from build123d import *

# Parameters (mm, degrees)
BOSS_EXTRUDE1_DEPTH     = 12.7
FILLET1_R               = 9.525
CUT_EXTRUDE3_DEPTH      = 171.371755619
CUT_EXTRUDE3_DEPTH_BACK = 171.371755619
SKETCH2_R               = 5.55625


with BuildPart() as part:
    # Sketch1 → Boss-Extrude1 (new body)
    with BuildSketch(Plane(origin=(0, 0, 0), x_dir=(0, 0, -1), z_dir=(1, 0, 0))):
        Polygon((0, 152.4), (-91.160761442, 0), (91.160761442, 0), align=None)
    extrude(amount=BOSS_EXTRUDE1_DEPTH)

    # Fillet1
    fillet1_edges = [part.edges().sort_by_distance(p)[0] for p in [
        (6.35, 152.4, 0),
    ]]
    fillet(fillet1_edges, radius=FILLET1_R)

    # Sketch2 → Cut-Extrude3 (cut, two sides: drawn at the far end of the back side and taken through both)
    with BuildSketch(Plane(origin=(0, 0, 0), x_dir=(0, 0, -1), z_dir=(1, 0, 0)).offset(-CUT_EXTRUDE3_DEPTH_BACK)):
        with Locations((0, 106.68)):
            Circle(SKETCH2_R)
    extrude(amount=CUT_EXTRUDE3_DEPTH + CUT_EXTRUDE3_DEPTH_BACK, mode=Mode.SUBTRACT)


solid = part.part
Here's how the part is built. I have some questions about the finished solid (model axes, mm). Coordinates: 2 decimals unless noted, no trailing zeros. Loops run counter-clockwise (first coordinate to the right, second up) from the corner with the lowest first, then second, coordinate; pieces in that order, holes last.
1. Imagine slicing it at A-A, the plane z = 0. Please give me the cut outline in (x, y).
2. I need wall thicknesses on L1, parallel to Y at x = 8.25, z = 0; L2, parallel to Z at x = 11.5, y = 107; L3, parallel to Z at x = 3, y = 106.5. Which ranges of each line are inside material? Lowest first, please.
3. Imagine slicing it at C-C, the plane y = 106.68. Please give me the cut outline in (x, z), and give its area (3 significant figures).
4. For P1, Ø1, axis at x = 7, y = 58, coming from the +Z side; P2, Ø3, axis at x = 6.5, z = 56, coming from the +Y side; P3, Ø6, axis at x = 4, z = 35, coming from the +Y side, each with a flat end and sliding along its axis, tell me the tip position at first contact or that it passes through.
5. Imagine slicing it at D-D, the plane y = 35.5. Please give me the cut outline in (x, z), and give its area (3 significant figures).
Taken from the geometry:
1. outline: (0, 0) - (12.7, 0) - (12.7, 101.12) - (0, 101.12) - close; (0, 112.24) - (12.7, 112.24) - (12.7, 143.37) - (0, 143.37) - close
2. L1: y = 0 to 101.12, 112.24 to 143.37
2. L2: z = -27.16 to -5.55, 5.55 to 27.16
2. L3: z = -27.46 to -5.55, 5.55 to 27.46
3. outline: (0, -27.35) - (12.7, -27.35) - (12.7, -5.56) - (0, -5.56) - close; (0, 5.56) - (12.7, 5.56) - (12.7, 27.35) - (0, 27.35) - close
3. area: 554 mm2
4. P1: stops at z = 56.77
4. P2: stops at y = 61.29
4. P3: stops at y = 98.9
5. outline: (0, -69.93) - (12.7, -69.93) - (12.7, 69.93) - (0, 69.93) - close
5. area: 1,780 mm2
